Geometry: final body of the model. Coordinates: model frame, mm. Face numbers are marked on the shaded views. A direction names the side the tool comes from. Coordinates: 2 decimals unless noted, no trailing zeros. Loops run counter-clockwise (first coordinate to the right, second up) from the corner with the lowest first, then second, coordinate; pieces in that order, holes last. Notation, with made-up numbers: M -18.5,44 L 22.5,44 A22 cw 22.5,59 Z; hole C -16,62.5 d6. An arc over 180 degrees is marked long. Write each question's results on one line, items separated by ' | '. Start each with the question number.
from build123d import *

# Parameters (mm, degrees)
SKETCH1_R           = 4.65
BOSS_EXTRUDE1_DEPTH = 12
SKETCH2_R           = 17.5
BOSS_EXTRUDE2_DEPTH = 2
SKETCH3_W           = 5
SKETCH3_H           = 13
BOSS_EXTRUDE3_DEPTH = 12
FILLET1_R           = 4
FILLET2_R           = 4
CUT_EXTRUDE1_DEPTH  = 29.434134416
SKETCH5_R           = 2.05
CUT_EXTRUDE2_DEPTH  = 70
FILLET3_R           = 4
SKETCH6_R           = 4.65
CUT_EXTRUDE3_DEPTH  = 33.897568299


with BuildPart() as part:
    # Sketch1 → Boss-Extrude1 (new body)
    with BuildSketch(Plane(origin=(0, 0, 0), x_dir=(1, 0, 0), z_dir=(0, 1, 0))):
        with Locations(Location((0, 0, 0), (0, 0, 270))):
            Circle(SKETCH1_R)
    extrude(amount=BOSS_EXTRUDE1_DEPTH)

    # Sketch2 → Boss-Extrude2 (add)
    with BuildSketch(Plane(origin=(0, 12, 0), x_dir=(1, 0, 0), z_dir=(0, 1, 0))):
        with Locations(Location((0, 0, 0), (0, 0, 270))):
            Circle(SKETCH2_R)
    extrude(amount=BOSS_EXTRUDE2_DEPTH)

    # Sketch3 → Boss-Extrude3 (add)
    with BuildSketch(Plane(origin=(0, 14, 0), x_dir=(1, 0, 0), z_dir=(0, 1, 0))):
        with Locations((7.5, 0)):
            Rectangle(SKETCH3_W, SKETCH3_H)
    boss_extrude3 = extrude(amount=BOSS_EXTRUDE3_DEPTH)

    # Mirror1: Boss-Extrude3 across plane
    add(boss_extrude3.mirror(Plane(origin=(0, 0, 0), x_dir=(0, 0, 1), z_dir=(1, 0, 0))))

    # Fillet1
    fillet1_edges = [part.edges().sort_by_distance(p)[0] for p in [
        (7.5, 26, -6.5),
        (7.5, 26, 6.5),
        (-7.5, 26, 6.5),
        (-7.5, 26, -6.5),
    ]]
    fillet(fillet1_edges, radius=FILLET1_R)

    # Fillet2
    fillet2_edges = [part.edges().sort_by_distance(p)[0] for p in [
        (7.5, 14, 6.5),
        (7.5, 14, -6.5),
        (-7.5, 14, -6.5),
        (-7.5, 14, 6.5),
    ]]
    fillet(fillet2_edges, radius=FILLET2_R)

    # Sketch4 → Cut-Extrude1 (cut, through all)
    with BuildSketch(Plane(origin=(0, 14, 0), x_dir=(1, 0, 0), z_dir=(0, 1, 0))):
        with BuildLine():
            Line((10, 14.361406616), (10, 0))
            Line((10, 0), (10, -14.361406616))
            ThreePointArc((10, -14.361406616), (15.512092057, -8.100925873), (17.5, 0))
            ThreePointArc((17.5, 0), (15.512092057, 8.100925873), (10, 14.361406616))
        make_face()
    cut_extrude1 = extrude(amount=-CUT_EXTRUDE1_DEPTH, mode=Mode.SUBTRACT)

    # Mirror2: Cut-Extrude1 across plane
    add(cut_extrude1.mirror(Plane(origin=(0, 0, 0), x_dir=(0, 0, 1), z_dir=(1, 0, 0))), mode=Mode.SUBTRACT)

    # Sketch5 → Cut-Extrude2 (cut)
    with BuildSketch(Plane(origin=(10, 0, 0), x_dir=(0, 0, -1), z_dir=(1, 0, 0))):
        with Locations((0, 20)):
            Circle(SKETCH5_R)
    extrude(amount=-CUT_EXTRUDE2_DEPTH, mode=Mode.SUBTRACT)

    # Fillet3
    fillet3_edges = [part.edges().sort_by_distance(p)[0] for p in [
        (10, 13, -14.361406616),
        (10, 13, 14.361406616),
        (-10, 13, 14.361406616),
        (-10, 13, -14.361406616),
    ]]
    fillet(fillet3_edges, radius=FILLET3_R)

    # Sketch6 → Cut-Extrude3 (cut, through all)
    with BuildSketch(Plane.XZ):
        with Locations(Location((0, 0, 0), (0, 0, 90))):
            Circle(SKETCH6_R)
    extrude(amount=-CUT_EXTRUDE3_DEPTH, mode=Mode.SUBTRACT)


solid = part.part
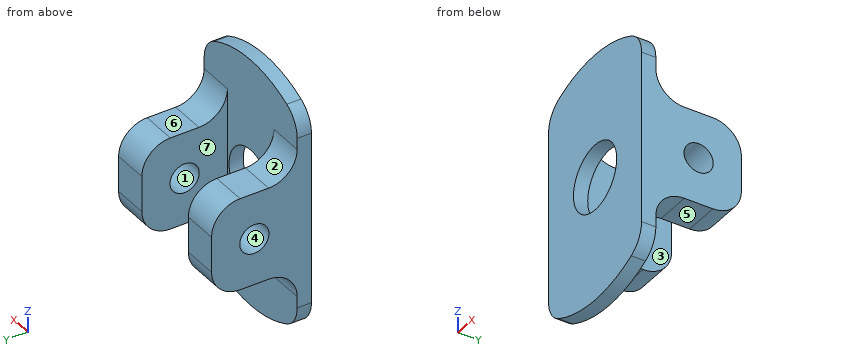
Item 1: Pull-direction query (Y, two-part tool) for the marked faces 1, 2, 3 and 4; classes: released by +Y, released by -Y, zero draft, split by the parting line, or undercut.
Item 2: Section D-D, the plane x = 0. Return loops of the section in (y, z), plus the area to 3 significant figures.
Item 3: Section A-A, the plane z = 0. Return loops of the section in (x, y).
Item 4: Section B-B, the plane y = 13.5. Return loops of the section in (x, z), plus the area to 3 significant figures.
Item 5: Contact query for flat-ended pins moving along their axis: P1, Ø4, axis at x = -5.5, z = 12.5, coming from the +Y side; P2, Ø5, axis at y = 21, z = -9.5, coming from the -X side (3 decimals); P3, Ø4.5, axis at x = 8, y = 20, coming from the -Z side; P4, Ø5.5, axis at y = 20, z = 0, coming from the +X side. Output: stop coordinate, or through.
Item 6: Section C-C, the plane y = 20. Return loops of the section in (x, z).
Item 7: Set-up query: the marked faces 5, 6 and 7. Return all of +Z, -Z, +X, -X, +Y, -Y with unobstructed straight access to the full face (end or side cutting, diameter ignored); none if empty.
Item 8: Ray query, L1, parallel to Y at x = 8.2, z = 0; L2, parallel to X at y = 13.25, z = 0; L3, parallel to Y at x = 4, z = 3.5. Return the intervals inside material, ascending. Write a range as [from, to].
Solutions:
1) face 1: undercut | face 2: released by +Y | face 3: zero draft | face 4: undercut
2) outline: M 12,-17.5 L 14,-17.5 L 14,-4.65 L 12,-4.65 Z; M 12,4.65 L 14,4.65 L 14,17.5 L 12,17.5 Z | area: 51.4 mm²
3) outline: M -10,12 L -4.65,12 L -4.65,14 L -5,14 L -5,17.95 L -10,17.95 Z; M -10,22.05 L -5,22.05 L -5,26 L -10,26 Z; M 4.65,12 L 10,12 L 10,17.95 L 5,17.95 L 5,14 L 4.65,14 Z; M 5,22.05 L 10,22.05 L 10,26 L 5,26 Z
4) outline: M -10,-12.09 A4 ccw -7.78,-15.68 A17.5 ccw 7.78,-15.68 A4 ccw 10,-12.09 L 10,12.09 A4 ccw 7.78,15.68 A17.5 ccw -7.78,15.68 A4 ccw -10,12.09 Z; hole C 0,0 d9.3 | area: 588 mm²
5) P1: stops at y = 14 | P2: passes through | P3: stops at z = -6.51 | P4: stops at x = 10
6) outline: M -10,-6.5 L -5,-6.5 L -5,-2.05 L -10,-2.05 Z; M -10,2.05 L -5,2.05 L -5,6.5 L -10,6.5 Z; M 5,-6.5 L 10,-6.5 L 10,-2.05 L 5,-2.05 Z; M 5,2.05 L 10,2.05 L 10,6.5 L 5,6.5 Z
7) face 5: -Z, +X, -X, +Y | face 6: +Z, +X, -X, +Y | face 7: +Z, -Z, +Y
8) L1: y = [12, 17.95], [22.05, 26] | L2: x = [-10, -4.65], [4.65, 10] | L3: y = [12, 14]
